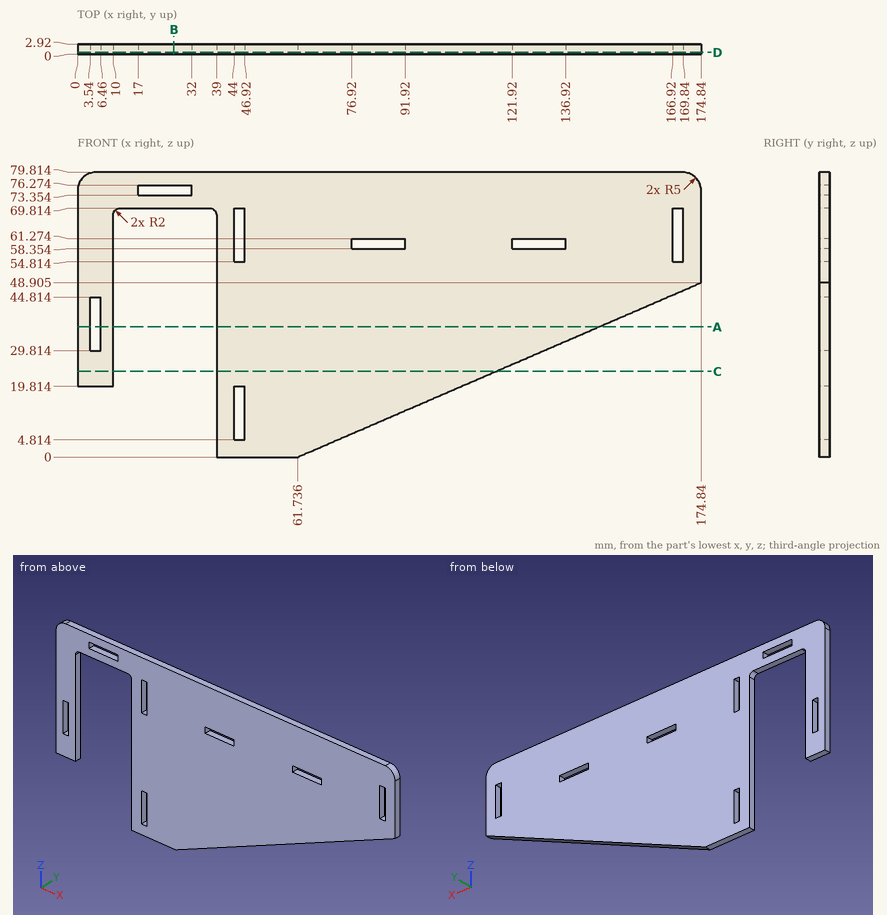
Job drawing, mm, ordinate dimensions from the low corner. One solid piece. Coordinates: 2 decimals unless noted, no trailing zeros. Write each loop counter-clockwise with the first axis right and the second up, starting at its lowest first coordinate (ties: lowest second). Pieces come first, ordered by that corner, then holes. Notation, with made-up numbers: (-30, 25.25) - (-21, 25.25) arc R23 ccw to (-21, 44.25) - close; hole circle Ø11 at (40, 14.5). An arc over 180 degrees is marked (long way). Use a Markdown table: item, result. Add a question column.
Item 1: Flat gauge pins, fed straight in: pin 1 (1.5 mm diameter, centred on x = 3, y = 1, fed in from -Z); pin 2 (1 mm diameter, centred on x = 150.5, y = 0.5, fed in from -Z) (1 decimal); pin 3 (1.5 mm diameter, centred on x = 30, y = 1, fed in from -Z). Where does each tip first touch, or does it go through?
Item 2: Band-saw the part on C-C, the plane z = 24. Give the cut face in (x, y).
Item 3: Band-saw the part on D-D, the plane y = 0.6. Give the number of separate pieces and of enclosed holes in the cut face, and give its area (3 significant figures).
Item 4: Band-saw the part on A-A, the plane z = 36.5. Give the cut face in (x, y).
Item 5: Drill centre lines: L1, parallel to X at y = 1.4, z = 60.5; L2, parallel to X at y = 0.5, z = 32.5; L3, parallel to X at y = 0.5, z = 55. Where is each one in solid material? Low to high. Write a range as from..to.
Item 6: Band-saw the part on B-B, the plane x = 27. Give the cut face in (y, z) (1 decimal).
Numbers:
| question | item | result |
|---|---|---|
| 1 | pin 1 | z = 19.81 |
| 1 | pin 2 | z = 38.2 |
| 1 | pin 3 | z = 69.81 |
| 2 | outline | (0, 0) - (10, 0) - (10, 2.92) - (0, 2.92) - close; (39, 0) - (117.24, 0) - (117.24, 2.92) - (39, 2.92) - close |
| 3 | separate pieces | 1 |
| 3 | enclosed holes | 7 |
| 3 | area | 8,650 mm2 |
| 4 | outline | (0, 0) - (3.54, 0) - (3.54, 2.92) - (0, 2.92) - close; (6.46, 0) - (10, 0) - (10, 2.92) - (6.46, 2.92) - close; (39, 0) - (146.15, 0) - (146.15, 2.92) - (39, 2.92) - close |
| 5 | L1 | 0..10, 39..44, 46.92..76.92, 91.92..121.92, 136.92..166.92, 169.84..174.84 |
| 5 | L2 | 0..3.54, 6.46..10, 39..136.9 |
| 5 | L3 | 0..10, 39..44, 46.92..166.92, 169.84..174.84 |
| 6 | outline | (0, 69.8) - (2.9, 69.8) - (2.9, 73.4) - (0, 73.4) - close; (0, 76.3) - (2.9, 76.3) - (2.9, 79.8) - (0, 79.8) - close |
